Check sheet for the drawn part. Datum: minimum x, y, z corner. Units: mm. Round coordinates to 2 decimals unless told otherwise and drop trailing zeros. Order: outer loops, then holes, each group sorted by start corner. A loop starts at its lowest first (then second) coordinate and runs counter-clockwise, first axis right, second up. Notation, with made-up numbers: M 76,28 L 111,28 A27 cw 111,54 Z; hole C 72.5,50 d4. An arc over 180 degrees is marked long. Answer as a JSON object with one key per item and string values. Group by question number.
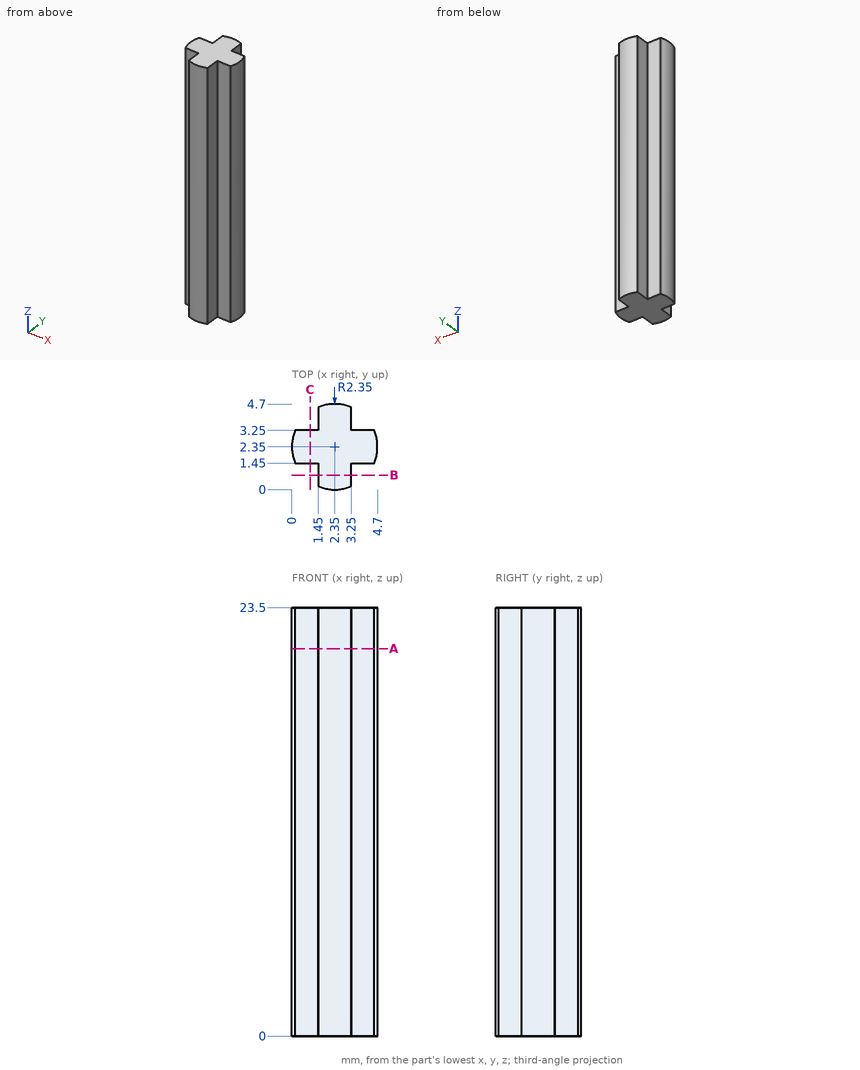
1) Thickness scan on line 1 along X through (y, z) = (3.65, 20.75); line 2 along Y through (x, z) = (2.5, 5.5). Record the ranges inside material, lowest first. Write a range as [from, to].
2) Sectioned sample at A-A (z = 21.25). Record the boundary of the cut face in (x, y), then the cut area to 3 significant figures.
3) Sectioned sample at B-B (y = 0.8). Record the boundary of the cut face in (x, z), then the cut area to 3 significant figures.
4) Go/stop test with flat-tipped pins: P1, Ø1, axis at y = 1.5, z = 16, coming from the -X side; P2, Ø1, axis at y = 4, z = 8, coming from the +X side; P3, Ø1.4, axis at x = 4, z = 14, coming from the -Y side. Record where each tip stops, or that it passes through.
Final values:
{
 "1": {"line 1": "x = [1.45, 3.25]", "line 2": "y = [0, 4.7]"},
 "2": {"outline": "M 0.18,1.45 L 1.45,1.45 L 1.45,0.18 A2.35 ccw 3.25,0.18 L 3.25,1.45 L 4.52,1.45 A2.35 ccw 4.52,3.25 L 3.25,3.25 L 3.25,4.52 A2.35 ccw 1.45,4.52 L 1.45,3.25 L 0.18,3.25 A2.35 ccw Z", "area": "13.3 mm^2"},
 "3": {"outline": "M 1.45,0 L 3.25,0 L 3.25,23.5 L 1.45,23.5 Z", "area": "42.3 mm^2"},
 "4": {"P1": "stops at x = 0.03", "P2": "stops at x = 3.25", "P3": "stops at y = 1.45"}
}
